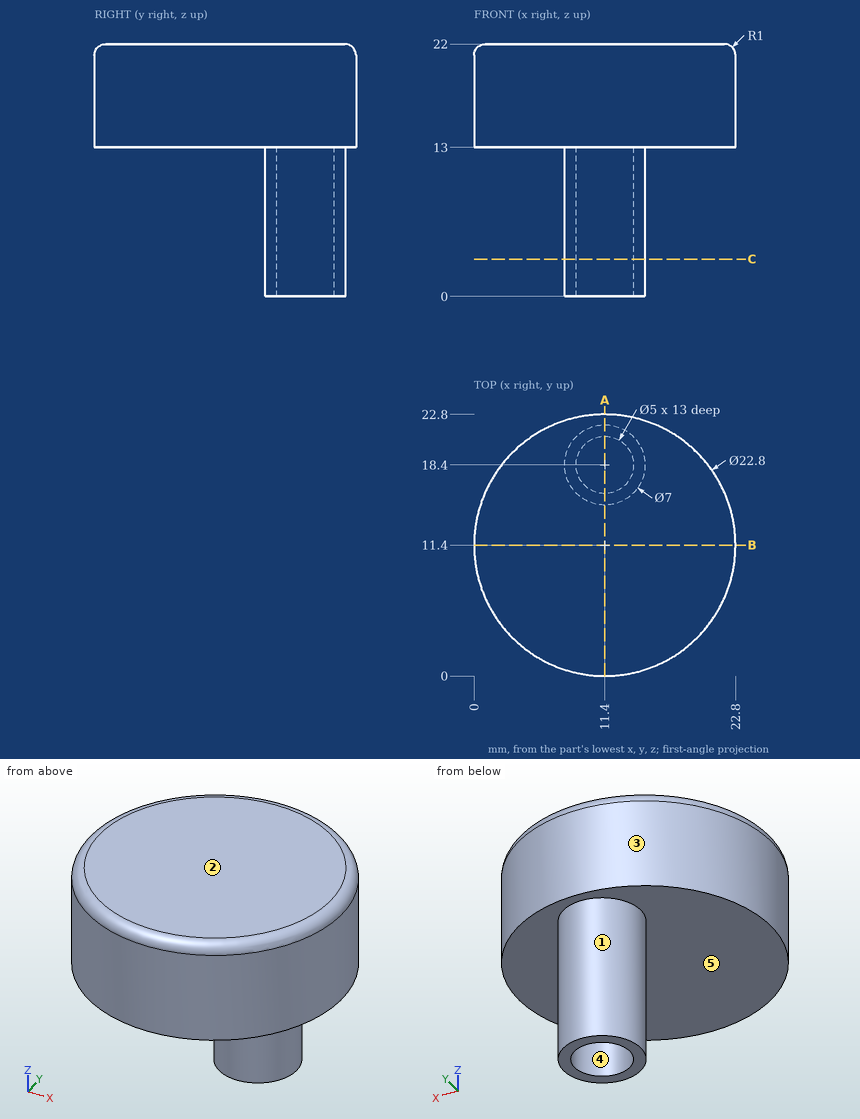
Part print with two shaded views. Sizes in mm from the minimum x, y, z corner. A direction names the side the tool comes from. Round coordinates to 2 decimals unless told otherwise and drop trailing zeros. Write each loop counter-clockwise with the first axis right and the second up, starting at its lowest first coordinate (ties: lowest second). Pieces come first, ordered by that corner, then holes. Notation, with made-up numbers: M 87,51 L 138,51 A12 cw 138,61 Z; hole C 30,43.25 d10. An arc over 180 degrees is marked long. Put each result on its own line as item: value. Start each with the question number.
1) Saw through at A-A, the plane x = 11.4. Write the cut outline in (y, z), and give its area (3 significant figures).
2) Drill centre lines: probe 1 along Y at (x, z) = (11.4, 5); probe 2 along X at (y, z) = (18.4, 7.75); probe 3 along Z at (x, y) = (9.25, 19). Where is each one in solid material? Low to high. Write a range as [from, to].
3) Pull direction X, two halves, no side cores. Call the marked faces 3, 4 and 5: pulls with the +X half, pulls with the -X half, needs draft (parallel to the pull), parting line crosses it, or undercut.
4) Saw through at B-B, the plane y = 11.4. Write the cut outline in (x, z).
5) 3-axis set-ups, long thin cutter, end or side, ignore diameter. For the marked faces 1 and 2: which of +Z, -Z, +X, -X, +Y, -Y reach the whole face in a straight line?
6) Saw through at C-C, the plane z = 3.25. Write the cut outline in (x, y), and give its area (3 significant figures).
7) Pin check, flat tips, straight feed: pin 1 Ø11.5 at (x, y) = (14, 7.5) entering from -Z; pin 2 Ø10 at (y, z) = (16.5, 13.5) entering from +X; pin 3 Ø5 at (y, z) = (5, 17.5) entering from -X; pin 4 Ø4 at (x, z) = (6, 11.5) entering from -Y. Stop position of each tip, or through.
Resolved:
1. outline: M 0,13 L 14.9,13 L 14.9,0 L 15.9,0 L 15.9,13 L 20.9,13 L 20.9,0 L 21.9,0 L 21.9,13 L 22.8,13 L 22.8,21 A1 ccw 21.8,22 L 1,22 A1 ccw 0,21 Z
1. area: 231 mm²
2. probe 1: [14.9, 15.9], [20.9, 21.9]
2. probe 2: [7.9, 8.9], [13.9, 14.9]
2. probe 3: [13, 22]
3. face 3: parting line crosses it
3. face 4: undercut
3. face 5: needs draft
4. outline: M 0,13 L 22.8,13 L 22.8,21 A1 ccw 21.8,22 L 1,22 A1 ccw 0,21 Z
5. face 1: -Z
5. face 2: +Z, +X, -X, +Y, -Y
6. outline: C 11.4,18.4 d7; hole C 11.4,18.4 d5
6. area: 18.8 mm²
7. pin 1: z = 13
7. pin 2: x = 22.8
7. pin 3: x = 0.69
7. pin 4: y = 0.75
